from build123d import *

# Parameters (mm, degrees)
EXTRUDE_1_DEPTH      = 9
EXTRUDE_1_DEPTH_BACK = 18
SKETCH_1_W           = 94
SKETCH_1_H           = 60.24
SKETCH_1_3_R         = 1.6
EXTRUDE_2_DEPTH      = 1.6
SKETCH_2_R           = 1.6
EXTRUDE_3_DEPTH      = 1.6
FILLET_1_R           = 3
SKETCH_3_W           = 42.24
SKETCH_3_H           = 14.8
CUT_EXTRUDE_1_DEPTH  = 4
SKETCH_4_W           = 42.24
SKETCH_4_H           = 14.8
CUT_EXTRUDE_2_DEPTH  = 4
SKETCH_5_W           = 76
SKETCH_5_H           = 14.8
CUT_EXTRUDE_3_DEPTH  = 4
SKETCH_6_W           = 76
SKETCH_6_H           = 14.8
CUT_EXTRUDE_4_DEPTH  = 4
FILLET_2_R           = 1
SKETCH_8_W           = 3
SKETCH_8_H           = 14.8
CUT_EXTRUDE_5_DEPTH  = 4
FILLET_3_R           = 1
SKETCH_9_W           = 31.32633541
SKETCH_9_H           = 1.6
CUT_EXTRUDE_6_DEPTH  = 4
FILLET_5_R           = 0.8


with BuildPart() as part:
    # 草图1 → 凸台-拉伸1 (new, two sides: drawn at the far end of the back side and taken through both)
    with BuildSketch(Plane(origin=(0, 0, 0), x_dir=(1, 0, 0), z_dir=(0, 1, 0)).offset(-EXTRUDE_1_DEPTH_BACK)):
        Rectangle(SKETCH_1_W, SKETCH_1_H)
        Polygon((-43, 15.663167705), (-43, 26.12), (-32.543167705, 26.12), (32.543167705, 26.12), (43, 26.12), (43, 15.663167705), (43, -15.663167705), (43, -26.12), (32.543167705, -26.12), (-32.543167705, -26.12), (-43, -26.12), (-43, -15.663167705), align=None, mode=Mode.SUBTRACT)
    extrude(amount=EXTRUDE_1_DEPTH + EXTRUDE_1_DEPTH_BACK)

    # 草图1<3> → 凸台-拉伸2 (add)
    # profile 1 of 4: a face of its own
    with BuildSketch(Plane(origin=(0, 0, 0), x_dir=(1, 0, 0), z_dir=(0, 1, 0))):
        with BuildLine():
            Line((-32.543167705, 26.12), (-43, 26.12))
            Line((-43, 26.12), (-43, 15.663167705))
            ThreePointArc((-43, 15.663167705), (-36.393398282, 19.513398282), (-32.543167705, 26.12))
        make_face()
        with Locations(Location((-39.3, 21.79, 0), (0, 0, 270))):
            Circle(SKETCH_1_3_R, mode=Mode.SUBTRACT)
    # profile 2 of 4: a face of its own
    with BuildSketch(Plane(origin=(0, 0, 0), x_dir=(1, 0, 0), z_dir=(0, 1, 0))):
        with BuildLine():
            Line((32.543167705, 26.12), (43, 26.12))
            Line((43, 26.12), (43, 15.663167705))
            ThreePointArc((43, 15.663167705), (36.393398282, 19.513398282), (32.543167705, 26.12))
        make_face()
        with Locations(Location((39.3, 21.79, 0), (0, 0, 270))):
            Circle(SKETCH_1_3_R, mode=Mode.SUBTRACT)
    # profile 3 of 4: a face of its own
    with BuildSketch(Plane(origin=(0, 0, 0), x_dir=(1, 0, 0), z_dir=(0, 1, 0))):
        with BuildLine():
            Line((43, -15.663167705), (43, -26.12))
            Line((43, -26.12), (32.543167705, -26.12))
            ThreePointArc((32.543167705, -26.12), (36.393398282, -19.513398282), (43, -15.663167705))
        make_face()
        with Locations(Location((39.3, -21.79, 0), (0, 0, 270))):
            Circle(SKETCH_1_3_R, mode=Mode.SUBTRACT)
    # profile 4 of 4: a face of its own
    with BuildSketch(Plane(origin=(0, 0, 0), x_dir=(1, 0, 0), z_dir=(0, 1, 0))):
        with BuildLine():
            ThreePointArc((-32.543167705, -26.12), (-36.393398282, -19.513398282), (-43, -15.663167705))
            Line((-43, -15.663167705), (-43, -26.12))
            Line((-43, -26.12), (-32.543167705, -26.12))
        make_face()
        with Locations(Location((-39.3, -21.79, 0), (0, 0, 270))):
            Circle(SKETCH_1_3_R, mode=Mode.SUBTRACT)
    extrude(amount=EXTRUDE_2_DEPTH)

    # 草图2 → 凸台-拉伸3 (add)
    # profile 1 of 4: a face of its own
    with BuildSketch(Plane(origin=(0, -18, 0), x_dir=(-1, 0, 0), z_dir=(0, -1, 0))):
        with BuildLine():
            Line((-43, 26.12), (-43, 12.570071225))
            ThreePointArc((-43, 12.570071225), (-34.272077939, 17.392077939), (-29.450071225, 26.12))
            Line((-29.450071225, 26.12), (-43, 26.12))
        make_face()
        with Locations(Location((-36, 21, 0), (0, 0, 90))):
            Circle(SKETCH_2_R, mode=Mode.SUBTRACT)
    # profile 2 of 4: a face of its own
    with BuildSketch(Plane(origin=(0, -18, 0), x_dir=(-1, 0, 0), z_dir=(0, -1, 0))):
        with BuildLine():
            Line((16.416573998, 26.12), (31.641993825, 26.12))
            add(Edge.make_bspline(
                [(16.416573998, 26.12), (24.309284633, -12.12635511), (31.641993825, 26.12)],
                knots=[1.876324373, 1.876324373, 1.876324373, 4.392355682, 4.392355682, 4.392355682], degree=2, weights=[1, 0.307705581, 1]))
        make_face()
        with Locations(Location((24, 21, 0), (0, 0, 90))):
            Circle(SKETCH_2_R, mode=Mode.SUBTRACT)
    # profile 3 of 4: a face of its own
    with BuildSketch(Plane(origin=(0, -18, 0), x_dir=(-1, 0, 0), z_dir=(0, -1, 0))):
        with BuildLine():
            Line((43, -12.570071225), (43, -26.12))
            Line((43, -26.12), (29.450071225, -26.12))
            ThreePointArc((29.450071225, -26.12), (34.272077939, -17.392077939), (43, -12.570071225))
        make_face()
        with Locations(Location((36, -21, 0), (0, 0, 90))):
            Circle(SKETCH_2_R, mode=Mode.SUBTRACT)
    # profile 4 of 4: a face of its own
    with BuildSketch(Plane(origin=(0, -18, 0), x_dir=(-1, 0, 0), z_dir=(0, -1, 0))):
        with BuildLine():
            Line((-43, -26.12), (-29.450071225, -26.12))
            ThreePointArc((-29.450071225, -26.12), (-34.272077939, -17.392077939), (-43, -12.570071225))
            Line((-43, -12.570071225), (-43, -26.12))
        make_face()
        with Locations(Location((-36, -21, 0), (0, 0, 90))):
            Circle(SKETCH_2_R, mode=Mode.SUBTRACT)
    extrude(amount=-EXTRUDE_3_DEPTH)

    # 圆角1
    fillet_1_edges = [part.edges().sort_by_distance(p)[0] for p in [
        (47, -4.5, 30.12),
        (-47, -4.5, 30.12),
        (-47, -4.5, -30.12),
        (47, -4.5, -30.12),
    ]]
    fillet(fillet_1_edges, radius=FILLET_1_R)

    # 草图3 → 切除-拉伸1 (cut)
    with BuildSketch(Plane.ZY.offset(47)):
        with Locations((0, -7.4)):
            Rectangle(SKETCH_3_W, SKETCH_3_H)
    extrude(amount=-CUT_EXTRUDE_1_DEPTH, mode=Mode.SUBTRACT)

    # 草图4 → 切除-拉伸2 (cut)
    with BuildSketch(Plane(origin=(47, 0, 0), x_dir=(0, 0, -1), z_dir=(1, 0, 0))):
        with Locations((0, -7.4)):
            Rectangle(SKETCH_4_W, SKETCH_4_H)
    extrude(amount=-CUT_EXTRUDE_2_DEPTH, mode=Mode.SUBTRACT)

    # 草图5 → 切除-拉伸3 (cut)
    with BuildSketch(Plane.XY.offset(30.12)):
        with Locations((0, -7.4)):
            Rectangle(SKETCH_5_W, SKETCH_5_H)
    extrude(amount=-CUT_EXTRUDE_3_DEPTH, mode=Mode.SUBTRACT)

    # 草图6 → 切除-拉伸4 (cut)
    with BuildSketch(Plane(origin=(0, 0, -30.12), x_dir=(-1, 0, 0), z_dir=(0, 0, -1))):
        with Locations((0, -7.4)):
            Rectangle(SKETCH_6_W, SKETCH_6_H)
    extrude(amount=-CUT_EXTRUDE_4_DEPTH, mode=Mode.SUBTRACT)

    # 圆角2
    fillet_2_edges = [part.edges().sort_by_distance(p)[0] for p in [
        (-45, 0, 21.12),
        (-45, -14.8, 21.12),
        (45, 0, -21.12),
        (45, -14.8, -21.12),
        (45, -14.8, 21.12),
        (45, 0, 21.12),
        (38, 0, 28.12),
        (38, -14.8, 28.12),
        (-38, -14.8, 28.12),
        (-38, 0, 28.12),
        (-38, 0, -28.12),
        (-38, -14.8, -28.12),
        (38, -14.8, -28.12),
        (38, 0, -28.12),
    ]]
    fillet(fillet_2_edges, radius=FILLET_2_R)

    # 草图8 → 切除-拉伸5 (cut)
    with BuildSketch(Plane.ZY.offset(47)):
        with Locations((-22.62, -7.4)):
            Rectangle(SKETCH_8_W, SKETCH_8_H)
    extrude(amount=-CUT_EXTRUDE_5_DEPTH, mode=Mode.SUBTRACT)

    # 圆角3
    fillet_3_edges = [part.edges().sort_by_distance(p)[0] for p in [
        (-45, -14.8, -24.12),
        (-45, 0, -24.12),
    ]]
    fillet(fillet_3_edges, radius=FILLET_3_R)

    # 草图9 → 切除-拉伸6 (cut)
    with BuildSketch(Plane(origin=(47, 0, 0), x_dir=(0, 0, -1), z_dir=(1, 0, 0))):
        with Locations((0, 0.8)):
            Rectangle(SKETCH_9_W, SKETCH_9_H)
    extrude(amount=-CUT_EXTRUDE_6_DEPTH, mode=Mode.SUBTRACT)

    # 圆角5
    # the kernel refuses this fillet: 0.8 mm, written as the material it adds along each edge
    with BuildSketch(Plane(origin=(47, 1.6, 15.663167705), x_dir=(0, -1, 0), z_dir=(-1, 0, 0))) as fillet_5_piece_1:
        with BuildLine():
            CenterArc((FILLET_5_R, -FILLET_5_R), FILLET_5_R, 90, 90)
            Line((0, -FILLET_5_R), (0, 0))
            Line((0, 0), (FILLET_5_R, 0))
        make_face()
    extrude(amount=4)
    with BuildSketch(Plane(origin=(47, 1.6, -15.663167705), x_dir=(0, -1, 0), z_dir=(-1, 0, 0))) as fillet_5_piece_2:
        with BuildLine():
            CenterArc((FILLET_5_R, FILLET_5_R), FILLET_5_R, 180, 90)
            Line((0, FILLET_5_R), (0, 0))
            Line((0, 0), (FILLET_5_R, 0))
        make_face()
    extrude(amount=4)
    # the kernel refuses this fillet: 0.8 mm, written as the material it takes off along each edge
    with BuildSketch(Plane(origin=(49, 0, -15.663167705), x_dir=(0, 0, -1), z_dir=(-1, 0, 0))) as fillet_5_2_piece_1:
        with BuildLine():
            CenterArc((FILLET_5_R, -FILLET_5_R), FILLET_5_R, 90, 90)
            Line((0, -FILLET_5_R), (0, 0))
            Line((0, 0), (FILLET_5_R, 0))
        make_face()
    extrude(amount=9.4, mode=Mode.SUBTRACT)
    with BuildSketch(Plane(origin=(49, 0, 15.663167705), x_dir=(0, 0, 1), z_dir=(-1, 0, 0))) as fillet_5_2_piece_2:
        with BuildLine():
            CenterArc((FILLET_5_R, FILLET_5_R), FILLET_5_R, 180, 90)
            Line((0, FILLET_5_R), (0, 0))
            Line((0, 0), (FILLET_5_R, 0))
        make_face()
    extrude(amount=9.4, mode=Mode.SUBTRACT)


solid = part.part
Could you check a few things on this model? Use its own coordinates, in mm. A direction names the side the tool comes from. Give positions to 0.01 mm unless a question says otherwise; leave off trailing zeros. Loops run counter-clockwise (first coordinate to the right, second up) from the corner with the lowest first, then second, coordinate; pieces in that order, holes last. Notation, with made-up numbers: M 70,63 L 81,63 A26 cw 81,97 Z; hole C 5,32 d5. An arc over 180 degrees is marked long. Answer as a JSON object with one key per item and string values.
Q1. Suppose I cut it at D-D, the plane y = -10. List the corners of the cut face in (x, z) for me, plus the area to 3 significant figures.
Values found:
{"outline": "M -47,-27.12 A3 ccw -44,-30.12 L -38,-30.12 L -38,-26.12 L -43,-26.12 L -43,-24.12 L -47,-24.12 Z; M -47,21.12 L -43,21.12 L -43,26.12 L -38,26.12 L -38,30.12 L -44,30.12 A3 ccw -47,27.12 Z; M 38,-30.12 L 44,-30.12 A3 ccw 47,-27.12 L 47,-21.12 L 43,-21.12 L 43,-26.12 L 38,-26.12 Z; M 38,26.12 L 43,26.12 L 43,21.12 L 47,21.12 L 47,27.12 A3 ccw 44,30.12 L 38,30.12 Z", "area": "204 mm²"}
Q2. If we mould it in two halves opening along Z, with no side actions, what happens to faces 5 (the cylindrical face through (-46.14, -4.31, -29.22)), 6 (the cylindrical face through (34.172, -17.211, 17.492)), 7 (the flat face through (-38, -7, 28))? For each: pulls with the +Z half, pulls with the -Z half, needs draft (parallel to the pull), parting line crosses it, or undercut.
Values found:
{"face 5": "pulls with the -Z half", "face 6": "undercut", "face 7": "needs draft"}
Q3. If I drill on probe 1 along X at (y, z) = (-12, 27); probe 2 along Y at (x, z) = (6, -27); probe 3 along X at (y, z) = (-16, -19.5), over which ranges is the centre line in solid material (lowest first)? Write a range as [from, to].
Values found:
{"probe 1": "x = [-47, -38], [38, 47]", "probe 2": "y = [-18, -14.8], [0, 9]", "probe 3": "x = [-47, -43], [43, 47]"}
Q4. Suppose I cut it at C-C, the plane x = 9. List the corners of the cut face in (y, z) for me.
Values found:
{"outline": "M -18,-30.12 L -14.8,-30.12 L -14.8,-26.12 L -18,-26.12 Z; M -18,26.12 L -14.8,26.12 L -14.8,30.12 L -18,30.12 Z; M 0,-30.12 L 9,-30.12 L 9,-26.12 L 0,-26.12 Z; M 0,26.12 L 9,26.12 L 9,30.12 L 0,30.12 Z"}
Q5. For faces 1 (the cylindrical face through (-36.47, 0.79, -19.44)), 2 (the flat face through (38, -7, 28)), 3 (the flat face through (-38, 1.6, 23)), 4 (the flat face through (45, -14.8, 0)), which set-ups out of +Z, -Z, +X, -X, +Y, -Y let a thin tool reach every point of the face, with its end or its side?
Values found:
{"face 1": "+Y, -Y", "face 2": "+Z, -Z", "face 3": "+Y", "face 4": "+X, -X"}
Q6. Suppose I cut it at A-A, the plane z = -11. List the corners of the cut face in (x, y) for me.
Values found:
{"outline": "M -47,-18 L -43,-18 L -43,-14.8 L -47,-14.8 Z; M -47,0 L -43,0 L -43,9 L -47,9 Z; M 43,-18 L 47,-18 L 47,-14.8 L 43,-14.8 Z; M 43,1.6 L 47,1.6 L 47,9 L 43,9 Z"}
Q7. Suppose I cut it at B-B, the plane y = 4.75. List the corners of the cut face in (x, z) for me.
Values found:
{"outline": "M -47,-27.12 A3 ccw -44,-30.12 L 44,-30.12 A3 ccw 47,-27.12 L 47,27.12 A3 ccw 44,30.12 L -44,30.12 A3 ccw -47,27.12 Z; hole M -43,-26.12 L 43,-26.12 L 43,26.12 L -43,26.12 Z"}
Q8. For P1, Ø3, axis at x = -39.5, z = -21, coming from the +Y side; P2, Ø1.9, axis at x = -39.3, z = 21.79, coming from the +Y side; P3, Ø3, axis at y = -8.5, z = -29, coming from the +X side, each with a flat end and sliding along its axis, tell me the tip position at first contact or that it passes through.
Values found:
{"P1": "stops at y = 1.6", "P2": "stops at y = -16.4", "P3": "stops at x = 46.98"}
